Here's how the part is built. I have some questions about the finished solid (model axes, mm). A direction names the side the tool comes from. Coordinates: 2 decimals unless noted, no trailing zeros. Write each loop counter-clockwise with the first axis right and the second up, starting at its lowest first coordinate (ties: lowest second). Pieces come first, ordered by that corner, then holes. Notation, with made-up numbers: (41.25, 57) -> (55.25, 57) arc R10 cw to (55.25, 70) -> close; hole circle Ø9 at (6.5, 56). An arc over 180 degrees is marked (long way). Use a Markdown table: item, result. Add a question column.
Item 1: Imagine slicing it at D-D, the plane x = -9.25. Write out the boundary of the cut face in (y, z).
Item 2: Imagine slicing it at C-C, the plane y = 0. Write out the boundary of the cut face in (x, z).
Item 3: If I drill on line 1 along X through (y, z) = (6.25, -10); line 2 along Z through (x, y) = (2.7, -2.5); line 3 along Y through (x, z) = (3, 6), over which ranges is the centre line in solid material (lowest first)? Write a range as from..to.
Item 4: If we mould it in two halves opening along Z, with no side actions, what happens to faces 3 (the cylindrical face through (1.97, -11.99, -0.53)), 4 (the flat face through (2, 0, 0)), 5 (the flat face through (0, -0.2, -2.5))? For each: pulls with the +Z half, pulls with the -Z half, needs draft (parallel to the pull), parting line crosses it, or undercut.
Item 5: On a 3-axis mill with a long thin cutter (end or side, diameter ignored), from which of +Z, -Z, +X, -X, +Y, -Y can I reach the whole of each face in a straight line? I mean faces 1 (the cylindrical face through (3, -1, 0)), 2 (the cylindrical face through (2.5, -3.3, 0.6)). Say none if no direction works.
Item 6: Imagine slicing it at B-B, the plane y = 2.5. Write out the boundary of the cut face in (x, z), and give its area (3 significant figures).
Item 7: Imagine slicing it at A-A, the plane z = 0. Write out the boundary of the cut face in (x, y).
Item 8: Will these pins go through, and if not, where does the flat tip stop? pin 1 Ø2 at (y, z) = (6, 0.5) entering from -X; pin 2 Ø1 at (x, y) = (-6, -4) entering from -Z; pin 3 Ø1.6 at (y, z) = (0, 0) entering from +X; pin 4 Ø0.7 at (x, z) = (-8.5, 1) entering from +Y.
Autodesk Inventor part; units mm, degrees
ref_plane "YZ Plane" through (0, 0, 0) normal (1, 0, 0) x (0, 1, 0)
ref_plane "XZ Plane" through (0, 0, 0) normal (0, 1, 0) x (-1, 0, 0)
ref_plane "XY Plane" through (0, 0, 0) normal (0, 0, 1) x (1, 0, 0)
sketch "Sketch1" plane through (0, 0, 0) normal (1, 0, 0) x (0, 1, 0)
  circle A0 centre (0, 0) radius 12
  circle A1 centre (0, 0) radius 2.25
  line L0 (16, 0) -> (-16, 0) construction
  circle A2 centre (-2.5, 0) radius 1
  circle A3 centre (2.5, 0) radius 1
  line L1 (1.35, 1.8) -> (1.35, -1.8)
  circle A4 centre (2.5, 0) radius 1.25
  circle A5 centre (-2.5, 0) radius 1.25
  point P0 (-2.0625, 0.8992)
  point P1 (-2.0625, -0.8992)
  point P2 (-1.95, 1.1225)
  point P3 (-1.95, -1.1225)
  point P4 (1.35, -0.4899)
  point P5 (1.35, 0.4899)
  dimension "d0" = 24
  dimension "d1" = 4.5
  dimension "d2" = 2
  dimension "d3" = 2
  dimension "d9" = 2.5
  dimension "d10" = 2.5
extrude "Extrusion1" add sketch "Sketch1" along normal blind 4 contours A0 | A3 A1 A4 L1 | A1 A4 A3 | A4 L1 A1 | A1 L1 A4 | L1 A4 A1 A5 | L1 A4 | A5 A1 A2 | A1 A2 A5
extrude "Extrusion3" add sketch "Sketch1" against normal blind 15 contours L1 A4 A1 A5
fillet "Fillet2" radius 1 2 edges at (0, -3.5, 0) (0, 1.5, 0)
sketch "Sketch2" plane through (4, 0, 0) normal (1, 0, 0) x (0, 0, -1)
  circle A0 centre (0, 0) radius 1
  dimension "d15" = 2
extrude "Extrusion4" cut sketch "Sketch2" against normal blind 2
properties part number "engine_gear_connector"
Ans:
| question | item | result |
|---|---|---|
| 1 | outline | (-1.95, -1.12) arc R2.25 ccw to (1.35, -1.8) -> (1.35, -0.49) arc R1.25 cw to (1.35, 0.49) -> (1.35, 1.8) arc R2.25 ccw to (-1.95, 1.12) arc R1.25 cw to start |
| 2 | outline | (-15, -2.25) -> (0, -2.25) -> (0, -12) -> (4, -12) -> (4, -1) -> (2, -1) -> (2, 1) -> (4, 1) -> (4, 12) -> (0, 12) -> (0, 2.25) -> (-15, 2.25) -> close |
| 3 | line 1 | x = 0..4 |
| 3 | line 2 | z = -11.74..-1, 1..11.74 |
| 3 | line 3 | y = -10.39..10.39 |
| 4 | face 3 | parting line crosses it |
| 4 | face 4 | undercut |
| 4 | face 5 | needs draft |
| 5 | face 1 | +X |
| 5 | face 2 | +X, -X |
| 6 | outline | (0, -11.74) -> (4, -11.74) -> (4, -1) -> (1, -1) arc R1 ccw to (0, -2) -> close; (0, 2) arc R1 ccw to (1, 1) -> (4, 1) -> (4, 11.74) -> (0, 11.74) -> close |
| 6 | area | 85.5 mm^2 |
| 7 | outline | (-15, -1.25) -> (0.34, -1.25) arc R1 ccw to (1, -1.5) -> (4, -1.5) -> (4, -1) -> (2, -1) -> (2, 1) -> (4, 1) -> (4, 1.5) -> (1, 1.5) arc R1 ccw to (0.34, 1.25) -> (-15, 1.25) -> close; (0, -12) -> (4, -12) -> (4, -3.5) -> (1, -3.5) arc R1 ccw to (0, -4.5) -> close; (0, 4.5) arc R1 ccw to (1, 3.5) -> (4, 3.5) -> (4, 12) -> (0, 12) -> close |
| 8 | pin 1 | stops at x = 0 |
| 8 | pin 2 | passes through |
| 8 | pin 3 | stops at x = 2 |
| 8 | pin 4 | stops at y = 1.35 |
